```python
from build123d import *

# Parameters (mm, degrees)
SKETCH2_W               = 45
SKETCH2_H               = 70
SKETCH2_W_2             = 25
SKETCH2_H_2             = 50
BOSS_EXTRUDE2_DEPTH     = 10
CUT_EXTRUDE1_REACH      = 72
BOSS_EXTRUDE3_DEPTH     = 10
SKETCH6_R               = 3.65
BOSS_EXTRUDE4_DEPTH     = 16
BOSS_EXTRUDE5_DEPTH     = 10
BOSS_EXTRUDE8_DEPTH     = 8
SKETCH9_W               = 6
SKETCH9_H               = 22
CUT_EXTRUDE2_DEPTH      = 6
CUT_EXTRUDE3_DEPTH      = 15.5
CUT_EXTRUDE3_DEPTH_BACK = 31.5
SKETCH11_R              = 2.55
CUT_EXTRUDE4_DEPTH      = 13
CHAMFER1_SIZE           = 0.2
CHAMFER1_SIZE2          = 0.115470054
CHAMFER2_SIZE           = 0.5
CHAMFER2_SIZE2          = 0.288675135
FILLET1_R               = 2


with BuildPart() as part:
    # Sketch2 → Boss-Extrude2 (new body)
    with BuildSketch(Plane.XY):
        with Locations((0, 35)):
            Rectangle(SKETCH2_W, SKETCH2_H)
        with Locations((0, 35)):
            Rectangle(SKETCH2_W_2, SKETCH2_H_2, mode=Mode.SUBTRACT)
    extrude(amount=BOSS_EXTRUDE2_DEPTH)

    # Sketch3 → Cut-Extrude1 (cut, up to next)
    with BuildSketch(Plane(origin=(0, 70, 0), x_dir=(1, 0, 0), z_dir=(0, 1, 0)), mode=Mode.PRIVATE) as cut_extrude1_sk1:
        Polygon((-9.9, 0), (-9.9, -4), (-5, -4), (-5, -8), (5, -8), (5, -4), (9.9, -4), (9.9, 0), align=None)
    cut_extrude1_tool1 = extrude(cut_extrude1_sk1.sketch, amount=-CUT_EXTRUDE1_REACH, mode=Mode.PRIVATE) & part.part
    add(cut_extrude1_tool1.solids().sort_by_distance((0, 70, 3.342282))[0], mode=Mode.SUBTRACT)

    # Sketch4 → Boss-Extrude3 (add)
    with BuildSketch(Plane(origin=(0, 70, 0), x_dir=(1, 0, 0), z_dir=(0, 1, 0))):
        with BuildLine():
            Line((-12, -10), (12, -10))
            ThreePointArc((12, -10), (7.5, -11.5), (4.8, -15.4))
            ThreePointArc((4.8, -15.4), (0, -19), (-4.8, -15.4))
            ThreePointArc((-4.8, -15.4), (-7.5, -11.5), (-12, -10))
        make_face()
    extrude(amount=-BOSS_EXTRUDE3_DEPTH)

    # Sketch6 → Boss-Extrude4 (add)
    with BuildSketch(Plane(origin=(0, 70, 0), x_dir=(1, 0, 0), z_dir=(0, 1, 0))):
        with Locations((0, -13)):
            Circle(SKETCH6_R)
    extrude(amount=BOSS_EXTRUDE4_DEPTH)

    # Sketch7 → Boss-Extrude5 (add)
    with BuildSketch(Plane.XZ):
        with BuildLine():
            Line((-22.5, 10), (-22.5, 12.456100996))
            Line((-22.5, 12.456100996), (-15.693142744, 14.258664405))
            ThreePointArc((-15.693142744, 14.258664405), (-10.135286431, 15.948047702), (-4.714257706, 18.035206128))
            ThreePointArc((-4.714257706, 18.035206128), (0, 19), (4.714257706, 18.035206128))
            ThreePointArc((4.714257706, 18.035206128), (10.135286431, 15.948047702), (15.693142744, 14.258664405))
            Line((15.693142744, 14.258664405), (22.5, 12.456100996))
            Line((22.5, 12.456100996), (22.5, 10))
            Line((22.5, 10), (-22.5, 10))
        make_face()
    extrude(amount=-BOSS_EXTRUDE5_DEPTH)

    # Sketch8 → Boss-Extrude8 (add, symmetric)
    with BuildSketch(Plane(origin=(0, 0, 0), x_dir=(0, 0, -1), z_dir=(1, 0, 0))):
        Polygon((-19, 77), (-23, 77), (-23, 55), (-18.660254038, 55), (-10, 60), (-10, 70), (-8, 70), (-8, 77), (-10, 77), align=None)
    extrude(amount=BOSS_EXTRUDE8_DEPTH, both=True)

    # Sketch9 → Cut-Extrude2 (cut)
    with BuildSketch(Plane.XY.offset(23)):
        with Locations((0, 66)):
            Rectangle(SKETCH9_W, SKETCH9_H)
    extrude(amount=-CUT_EXTRUDE2_DEPTH, mode=Mode.SUBTRACT)

    # Sketch10 → Cut-Extrude3 (cut, two sides)
    with BuildSketch(Plane.ZY.offset(8)) as cut_extrude3_sk:
        with BuildLine():
            Line((18.35, 74.5), (18.35, 57.5))
            ThreePointArc((18.35, 57.5), (20, 55.85), (21.65, 57.5))
            Line((21.65, 57.5), (21.65, 74.5))
            ThreePointArc((21.65, 74.5), (20, 76.15), (18.35, 74.5))
        make_face()
    extrude(amount=CUT_EXTRUDE3_DEPTH, mode=Mode.SUBTRACT)
    extrude(cut_extrude3_sk.sketch, amount=-CUT_EXTRUDE3_DEPTH_BACK, mode=Mode.SUBTRACT)

    # Sketch11 → Cut-Extrude4 (cut)
    with BuildSketch(Plane(origin=(0, 86, 0), x_dir=(1, 0, 0), z_dir=(0, 1, 0))):
        with Locations((0, -13)):
            Circle(SKETCH11_R)
    extrude(amount=-CUT_EXTRUDE4_DEPTH, mode=Mode.SUBTRACT)

    # Chamfer1
    chamfer1_edges = [part.edges().sort_by_distance(p)[0] for p in [
        (-2.55, 86, 13),
    ]]
    chamfer1_side = [part.faces().sort_by_distance(p)[0] for p in [
        (-3.54676241, 86, 13),
    ]]
    chamfer(chamfer1_edges, length=CHAMFER1_SIZE, length2=CHAMFER1_SIZE2, reference=chamfer1_side[0])

    # Chamfer2
    chamfer2_edges = [part.edges().sort_by_distance(p)[0] for p in [
        (-3.65, 86, 13),
    ]]
    chamfer2_side = [part.faces().sort_by_distance(p)[0] for p in [
        (-3.65, 81.5, 13),
    ]]
    chamfer(chamfer2_edges, length=CHAMFER2_SIZE, length2=CHAMFER2_SIZE2, reference=chamfer2_side[0])

    # Fillet1
    fillet1_edges = [part.edges().sort_by_distance(p)[0] for p in [
        (-22.5, 70, 5),
        (22.5, 70, 5),
        (22.5, 0, 6.228050498),
        (-22.5, 0, 6.228050498),
    ]]
    fillet(fillet1_edges, radius=FILLET1_R)


solid = part.part
```
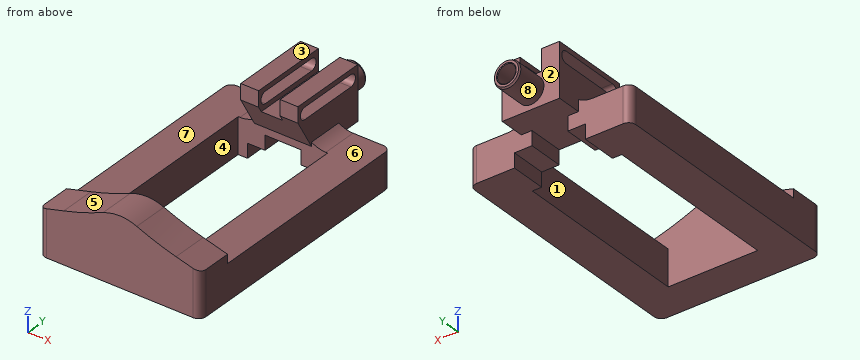
Build history of the part. All positions in model axes, mm. Face numbers are marked on the shaded views. A direction names the side the tool comes from. Round coordinates to 2 decimals unless told otherwise and drop trailing zeros. Write each loop counter-clockwise with the first axis right and the second up, starting at its lowest first coordinate (ties: lowest second). Pieces come first, ordered by that corner, then holes. Notation, with made-up numbers: (-25.75, 43) -> (31.25, 43) arc R23 ccw to (31.25, 62) -> close; hole circle Ø7 at (-7.5, -9.75). An arc over 180 degrees is marked (long way). Put each result on its own line as item: value.
Item 1: Slice it at A-A, the plane y = 12. Give the cut face in (x, z), plus the area to 3 significant figures.
Here are the results:
outline: (-22.5, 0) -> (-12.5, 0) -> (-12.5, 10) -> (-22.5, 10) -> close; (12.5, 0) -> (22.5, 0) -> (22.5, 10) -> (12.5, 10) -> close
area: 200 mm^2
Item 2: Two-plate mould, pull along Y, no slides. Class the marked faces 1, 2 and 3: pulls with the +Y half, pulls with the -Y half, needs draft (parallel to the pull), parting line crosses it, or undercut.
Here are the results:
face 1: undercut
face 2: pulls with the +Y half
face 3: needs draft
Item 3: Tool access for the marked faces 4, 5, 6, 7 and 8: list every direction of +Z, -Z, +X, -X, +Y, -Y with a clear straight run to the whole face (end or side of a thin tool).
Here are the results:
face 4: +Z, -Z
face 5: +Z, -X, -Y
face 6: +Z, +X, +Y
face 7: +Z, -X, +Y
face 8: +Y
Item 4: Slice it at C-C, the plane y = 66.5. Count the separate pieces of the cut face and the enclosed holes in it, plus the area to 3 significant figures.
Here are the results:
separate pieces: 3
enclosed holes: 0
area: 473 mm^2
Item 5: Wall check: probe 1 along X at (y, z) = (75.5, 13); probe 2 along Z at (x, y) = (0, 80); probe 3 along X at (y, z) = (63.5, 4.5). Give the ranges that are in metal, low to high. Write a range as from..to.
Here are the results:
probe 1: x = -8..-2.55, 2.55..8
probe 2: z = 9.35..10.45, 15.55..16.65
probe 3: x = -22.5..-5, 5..22.5
Item 6: Slice it at D-D, the plane x = 0. Give the cut face in (y, z), plus the area to 3 significant figures.
Here are the results:
outline: (0, 0) -> (10, 0) -> (10, 19) -> (0, 19) -> close; (55.96, 17) -> (60, 10) -> (60, 8) -> (77, 8) -> (77, 9.35) -> (85.5, 9.35) -> (86, 9.64) -> (86, 10.25) -> (85.88, 10.45) -> (73, 10.45) -> (73, 15.55) -> (85.88, 15.55) -> (86, 15.75) -> (86, 16.36) -> (85.5, 16.65) -> (77, 16.65) -> (77, 17) -> close
area: 356 mm^2
Item 7: Slice it at B-B, the plane z = 20. Give the cut face in (x, y), plus the area to 3 significant figures.
Here are the results:
outline: (-8, 55) -> (-3, 55) -> (-3, 55.85) -> (-8, 55.85) -> close; (-8, 76.15) -> (-3, 76.15) -> (-3, 77) -> (-8, 77) -> close; (3, 55) -> (8, 55) -> (8, 55.85) -> (3, 55.85) -> close; (3, 76.15) -> (8, 76.15) -> (8, 77) -> (3, 77) -> close
area: 17.0 mm^2
Item 8: Flat gauge pins, fed straight in: P1, Ø1, axis at x = 7, z = 18.5, coming from the -Y side; P2, Ø1.8, axis at x = -0.5, y = 63, coming from the +Z side; P3, Ø4, axis at x = 16.5, y = 59, coming from the +Z side. Where does each tip first touch, or does it go through?
Here are the results:
P1: stops at y = 55
P2: stops at z = 17
P3: stops at z = 10
